from build123d import *

# Parameters (mm, degrees)
SKETCH_1_W          = 27.5
SKETCH_1_H          = 25
SKETCH_1_W_2        = 21.5
SKETCH_1_H_2        = 19
EXTRUDE_1_DEPTH     = 36
SKETCH_3_W          = 15
SKETCH_3_H          = 30
CUT_EXTRUDE_1_DEPTH = 24.5
CUT_EXTRUDE_2_REACH = 55.397
SKETCH_4_W          = 7.5
SKETCH_4_H          = 24
SKETCH_5_W          = 25
SKETCH_5_H          = 3
SKETCH_5_H_2        = 3.5
CUT_EXTRUDE_3_DEPTH = 52.742149163
SKETCH_6_W          = 15
SKETCH_6_H          = 6.5
EXTRUDE_2_DEPTH     = 3
FILLET_1_R          = 1
SKETCH_7_W          = 1
SKETCH_7_H          = 25
CUT_EXTRUDE_5_DEPTH = 50.249365478
FILLET_3_R          = 1


with BuildPart() as part:
    # 草图1 → 凸台-拉伸1 (new body)
    with BuildSketch(Plane(origin=(0, 0, 0), x_dir=(1, 0, 0), z_dir=(0, 1, 0))):
        with Locations((16.75, 12.5)):
            Rectangle(SKETCH_1_W, SKETCH_1_H)
        with Locations((16.75, 12.5)):
            Rectangle(SKETCH_1_W_2, SKETCH_1_H_2, mode=Mode.SUBTRACT)
    extrude(amount=EXTRUDE_1_DEPTH)

    # 草图3 → 切除-拉伸1 (cut)
    with BuildSketch(Plane(origin=(30.5, 0, 0), x_dir=(0, 0, -1), z_dir=(1, 0, 0))):
        with Locations((12.5, 18)):
            Rectangle(SKETCH_3_W, SKETCH_3_H)
    extrude(amount=-CUT_EXTRUDE_1_DEPTH, mode=Mode.SUBTRACT)

    # 草图4 → 切除-拉伸2 (cut, up to next)
    with BuildSketch(Plane(origin=(0, 0, -25), x_dir=(-1, 0, 0), z_dir=(0, 0, -1)), mode=Mode.PRIVATE) as cut_extrude_2_sk1:
        with Locations((-12.75, 24)):
            Rectangle(SKETCH_4_W, SKETCH_4_H)
    cut_extrude_2_tool1 = extrude(cut_extrude_2_sk1.sketch, amount=-CUT_EXTRUDE_2_REACH, mode=Mode.PRIVATE) & part.part
    cut_extrude_2 = cut_extrude_2_tool1.solids().sort_by_distance((12.75, 24, -25))[0]
    add(cut_extrude_2, mode=Mode.SUBTRACT)

    # 草图5 → 切除-拉伸3 (cut, through all)
    with BuildSketch(Plane(origin=(30.5, 0, 0), x_dir=(0, 0, -1), z_dir=(1, 0, 0))):
        with Locations((12.5, 34.5)):
            Rectangle(SKETCH_5_W, SKETCH_5_H)
        with Locations((12.5, 1.75)):
            Rectangle(SKETCH_5_W, SKETCH_5_H_2)
    extrude(amount=-CUT_EXTRUDE_3_DEPTH, mode=Mode.SUBTRACT)

    # 草图6 → 凸台-拉伸2 (add)
    with BuildSketch(Plane(origin=(30.5, 0, 0), x_dir=(0, 0, -1), z_dir=(1, 0, 0))):
        with Locations((12.5, 17.75)):
            Rectangle(SKETCH_6_W, SKETCH_6_H)
    extrude(amount=-EXTRUDE_2_DEPTH)

    # 圆角1
    fillet_1_edges = [part.edges().sort_by_distance(p)[0] for p in [
        (30.5, 9, -5),
        (30.5, 27, -20),
        (27.5, 14.5, -12.5),
        (27.5, 21, -12.5),
        (30.5, 27, -5),
        (16.5, 33, -23.5),
        (30.5, 9, -20),
        (6, 18.25, -3),
        (27.5, 18.25, -3),
        (6, 18.25, -22),
        (27.5, 18.25, -22),
        (30.5, 18.25, 0),
        (3, 18.25, 0),
        (3, 18.25, -25),
        (30.5, 18.25, -25),
        (3, 33, -12.5),
        (9, 33, -23.5),
        (27.5, 33, -21),
        (27.5, 33, -4),
        (16.75, 33, -3),
        (6, 33, -12.5),
        (7.5, 33, -22),
        (22, 33, -22),
        (16.75, 33, 0),
        (3, 3.5, -12.5),
        (16.75, 3.5, 0),
        (16.75, 3.5, -25),
    ]]
    fillet(fillet_1_edges, radius=FILLET_1_R)

    # 草图7 → 切除-拉伸5 (cut, through all)
    with BuildSketch(Plane(origin=(0, 33, 0), x_dir=(1, 0, 0), z_dir=(0, 1, 0))):
        with Locations((3.5, 12.5)):
            Rectangle(SKETCH_7_W, SKETCH_7_H)
    extrude(amount=-CUT_EXTRUDE_5_DEPTH, mode=Mode.SUBTRACT)

    # 圆角3
    fillet_3_edges = [part.edges().sort_by_distance(p)[0] for p in [
        (4, 33, -13),
        (4, 18.75, -25),
        (4, 3.5, -12.5),
        (4, 18.25, 0),
        (4, 32.707106781, -0.292893219),
        (4, 3.792893219, -24.707106781),
        (4, 3.792893219, -0.292893219),
    ]]
    fillet(fillet_3_edges, radius=FILLET_3_R - 0.0001)  # a hair under: the kernel refuses the full size

    # 镜向1: 切除-拉伸2 across plane
    add(cut_extrude_2.mirror(Plane(origin=(0, 0, -12.5), x_dir=(1, 0, 0), z_dir=(0, 0, -1))), mode=Mode.SUBTRACT)


solid = part.part
Work out the finished part from the listing and answer in its coordinate system (mm). A direction names the side the tool comes from. Give positions to 0.01 mm unless a question says otherwise; leave off trailing zeros. Loops run counter-clockwise (first coordinate to the right, second up) from the corner with the lowest first, then second, coordinate; pieces in that order, holes last. Notation, with made-up numbers: (-32.75, -4.5) - (16.25, -4.5) arc R32 ccw to (16.25, 34.5) - close; hole circle Ø4 at (20.5, 17). An arc over 180 degrees is marked (long way). Answer in a Markdown table with one row per item.
(1) Section D-D (x = 23) is taken. Give the vertices of the cut face in (y, z).
Results list:
| item | result |
|---|---|
| outline | (3.5, -24) arc R1 ccw to (4.5, -25) - (33, -25) - (33, -23) arc R1 ccw to (32, -22) - (3.5, -22) - close; (3.5, -3) - (32, -3) arc R1 ccw to (33, -2) - (33, -1) arc R1 ccw to (32, 0) - (4.5, 0) arc R1 ccw to (3.5, -1) - close |
(2) For a pull along Z with two mould halves and no side action, classify faces 1 (the face through (6.972, 32.715, -0.301)), 2 (the face through (4.285, 3.801, -12.661)), 3 (the face through (21.43, 32.715, -2.699)), 4 (the face through (17.571, 3.785, -24.699)) as pulls with the +Z half, pulls with the -Z half, needs draft (parallel to the pull), parting line crosses it, or undercut.
Results list:
| item | result |
|---|---|
| face 1 | pulls with the +Z half |
| face 2 | needs draft |
| face 3 | undercut |
| face 4 | pulls with the -Z half |
(3) Section C-C (x = 11.5) is taken. Give the vertices of the cut face in (y, z).
Results list:
| item | result |
|---|---|
| outline | (3.5, -24) arc R1 ccw to (4.5, -25) - (12, -25) - (12, -22) - (3.5, -22) - close; (3.5, -3) - (12, -3) - (12, 0) - (4.5, 0) arc R1 ccw to (3.5, -1) - close |
(4) Section A-A (y = 30.5) is taken. State how many separate pieces and enclosed holes the cut face has, and give its area (3 significant figures).
Results list:
| item | result |
|---|---|
| separate pieces | 3 |
| enclosed holes | 0 |
| area | 164 mm² |
(5) Consider L1, parallel to Z at x = 21.5, y = 24; L2, parallel to X at y = 19.5, z = -8; L3, parallel to X at y = 13.25, z = -6.25. Determine where each line is inside the solid, lowest interval first. Write a range as [from, to].
Results list:
| item | result |
|---|---|
| L1 | z = [-25, -22], [-3, 0] |
| L2 | x = [4, 6], [27.5, 30.5] |
| L3 | x = [4, 6] |
(6) Flat-ended cylindrical pins translate along their axes: pin 1 Ø1 at (x, z) = (29.5, -10) entering from -Y; pin 2 Ø2 at (x, z) = (30, -8.5) entering from +Y; pin 3 Ø1.5 at (x, z) = (14, -23.5) entering from +Y. Find the tip coordinate at first contact, or state that the pin passes through.
Results list:
| item | result |
|---|---|
| pin 1 | stops at y = 14.5 |
| pin 2 | stops at y = 21 |
| pin 3 | stops at y = 12 |
(7) A tool of negligible diameter and unlimited length cuts with its end or side. For faces 5 (the face through (13, 12, -1)), 6 (the face through (30, 21, -12)), 7 (the face through (30.215, 9.077, -20.301)), 8 (the face through (27.785, 20.699, -12.605)), from which of +Z, -Z, +X, -X, +Y, -Y can it reach the whole face along a straight path? Write none if from no direction.
Results list:
| item | result |
|---|---|
| face 5 | +Z, -Z, +Y |
| face 6 | +X, +Y |
| face 7 | +X, -Y |
| face 8 | +Y |
